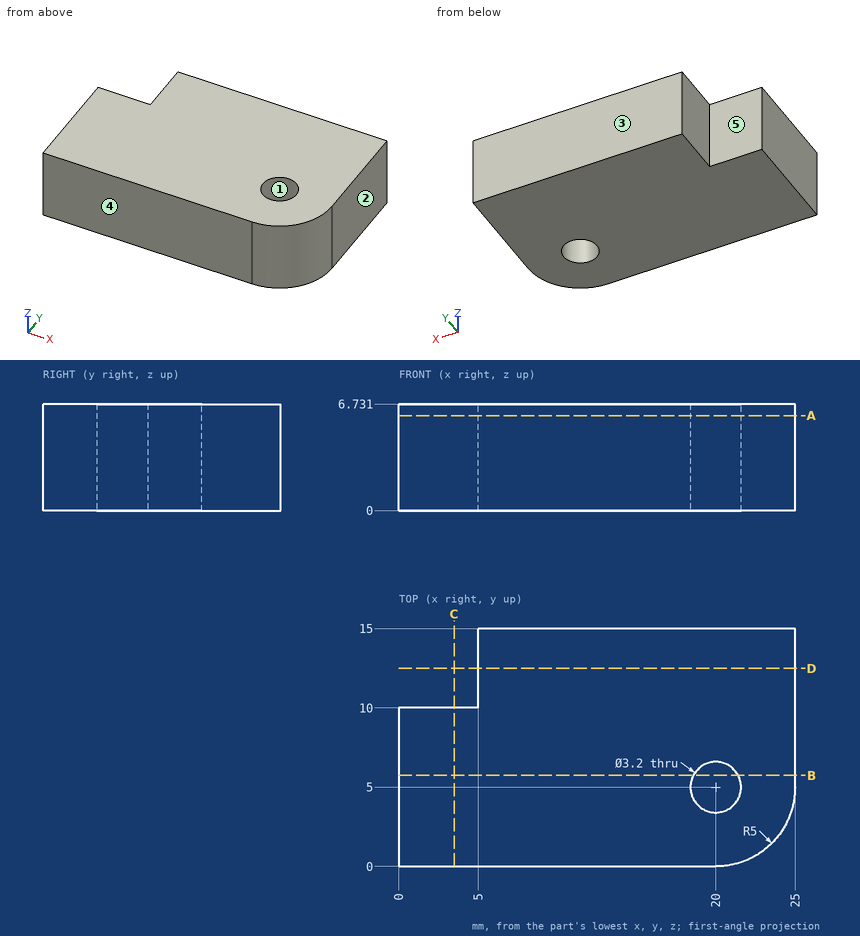
Study the drawing (mm; zero at the part's minimum x, y, z) and answer. A direction names the side the tool comes from. Coordinates: 2 decimals unless noted, no trailing zeros. Write each loop counter-clockwise with the first axis right and the second up, starting at its lowest first coordinate (ties: lowest second). Pieces come first, ordered by that corner, then holes. Notation, with made-up numbers: (64.5, 65.5) - (100.5, 65.5) arc R24 cw to (100.5, 92.5) - close; hole circle Ø8 at (-30.5, 35.5). An arc over 180 degrees is marked (long way). Return JSON: item names as keys, results as strings. Group by question number.
1. Determine the mould class of the marked faces 1, 2 and 3 for opening direction Y: released by +Y, released by -Y, zero draft, split by the parting line, or undercut.
2. Given pin 1 (1.5 mm diameter, centred on x = 1.5, z = 3.5, fed in from +Y); pin 2 (1.5 mm diameter, centred on y = 13, z = 4, fed in from -X), each flat-ended and moving along its own axis, determine where each tip first touches the part or whether it passes through.
3. A cutting plane is placed at A-A, the plane z = 6. Determine the outline of the cut face in (x, y), plus the area to 3 significant figures.
4. A cutting plane is placed at B-B, the plane y = 5.75. Determine the outline of the cut face in (x, z), plus the area to 3 significant figures.
5. Which of the six approach directions +Z, -Z, +X, -X, +Y, -Y give full straight-line access (tool end or side, diameter ignored) to the marked faces 4 and 5?
6. A cutting plane is placed at C-C, the plane x = 3.5. Determine the outline of the cut face in (y, z).
7. A cutting plane is placed at D-D, the plane y = 12.5. Determine the outline of the cut face in (x, z).
8. Straight lines are drawn through the part: L1, parallel to Y at x = 20, z = 2.25; L2, parallel to X at y = 13.5, z = 1; L3, parallel to X at y = 3.75, z = 3. For each, find the intervals that lie inside material, in ascending order.
Ans:
{
 "1": {"face 1": "undercut", "face 2": "zero draft", "face 3": "released by +Y"},
 "2": {"pin 1": "y = 10", "pin 2": "x = 5"},
 "3": {"outline": "(0, 0) - (20, 0) arc R5 ccw to (25, 5) - (25, 15) - (5, 15) - (5, 10) - (0, 10) - close; hole circle Ø3.2 at (20, 5)", "area": "337 mm²"},
 "4": {"outline": "(0, 0) - (18.59, 0) - (18.59, 6.73) - (0, 6.73) - close; (21.41, 0) - (25, 0) - (25, 6.73) - (21.41, 6.73) - close", "area": "149 mm²"},
 "5": {"face 4": "+Z, -Z, +X, -X, -Y", "face 5": "+Z, -Z, -X, +Y"},
 "6": {"outline": "(0, 0) - (10, 0) - (10, 6.73) - (0, 6.73) - close"},
 "7": {"outline": "(5, 0) - (25, 0) - (25, 6.73) - (5, 6.73) - close"},
 "8": {"L1": "0 to 3.4, 6.6 to 15", "L2": "5 to 25", "L3": "0 to 19, 21 to 24.84"}
}
